The model under review builds one solid part; all positions refer to its coordinate system, in mm. A direction names the side the tool comes from. Round coordinates to 2 decimals unless told otherwise and drop trailing zeros. Loops run counter-clockwise (first coordinate to the right, second up) from the corner with the lowest first, then second, coordinate; pieces in that order, holes last. Notation, with made-up numbers: M 18.25,21 L 73.25,21 A26 cw 73.25,59 Z; hole C 30.5,-13 d3. An arc over 180 degrees is marked long. Use a Markdown table: item, result. Add a question column.
```python
from build123d import *

# Parameters (mm, degrees)
SKETCH1_W                    = 76.2
SKETCH1_H                    = 88.9
BOSS_EXTRUDE1_DEPTH          = 1.27
CUT_EXTRUDE_THIN1_DEPTH      = 59.599181735
CUT_EXTRUDE_THIN1_DEPTH_BACK = 2.794
SKETCH3_W                    = 2.794
SKETCH3_H                    = 44.704
CHAMFER1_SIZE                = 0.254


with BuildPart() as part:
    # Sketch1 → Boss-Extrude1 (new, symmetric)
    with BuildSketch(Plane(origin=(0, 0, 0), x_dir=(1, 0, 0), z_dir=(0, 1, 0))):
        Rectangle(SKETCH1_W, SKETCH1_H)
    extrude(amount=BOSS_EXTRUDE1_DEPTH, both=True)

    # Sketch3 → Cut-Extrude-Thin1 (cut, two sides: drawn at the far end of the back side and taken through both)
    with BuildSketch(Plane(origin=(0, 1.27, 0), x_dir=(1, 0, 0), z_dir=(0, 1, 0)).offset(-CUT_EXTRUDE_THIN1_DEPTH_BACK)):
        with Locations((0, -22.098)):
            Rectangle(SKETCH3_W, SKETCH3_H)
    extrude(amount=CUT_EXTRUDE_THIN1_DEPTH + CUT_EXTRUDE_THIN1_DEPTH_BACK, mode=Mode.SUBTRACT)

    # Chamfer1
    chamfer1_edges = [part.edges().sort_by_distance(p)[0] for p in [
        (38.1, 1.27, 0),
        (19.7485, -1.27, 44.45),
        (0, -1.27, -0.254),
        (1.397, -1.27, 22.098),
        (-1.397, -1.27, 22.098),
        (0, 1.27, -44.45),
        (19.7485, 1.27, 44.45),
        (1.397, 1.27, 22.098),
        (0, 1.27, -0.254),
        (-1.397, 1.27, 22.098),
        (-38.1, 1.27, 0),
        (0, -1.27, -44.45),
        (38.1, -1.27, 0),
        (-19.7485, -1.27, 44.45),
        (-38.1, -1.27, 0),
        (-19.7485, 1.27, 44.45),
    ]]
    chamfer(chamfer1_edges, length=CHAMFER1_SIZE)


solid = part.part
```
(1) To check wall thickness, follow probe 1 along X at (y, z) = (0.5, 30.5); probe 2 along X at (y, z) = (-1.1, 18); probe 3 along Z at (x, y) = (-0.5, -1.1). State the ranges of each line that lie inside material, in increasing order.
(2) Consider section B-B, the plane y = -0.1. Give the boundary of the cut face in (x, z).
(3) Consider section A-A, the plane z = 17. Give the boundary of the cut face in (x, y), then the cut area to 3 significant figures.
(4) For faces 1 (the face through (38.1, 0, 1)), 2 (the face through (-1.397, 0, 22)), list the 3-axis set-ups (+Z, -Z, +X, -X, +Y, -Y) from which the entire face can be reached by the end or side of a thin tool; tool diameter is ignored.
Found:
| question | item | result |
|---|---|---|
| 1 | probe 1 | x = -38.1 to -1.4, 1.4 to 38.1 |
| 1 | probe 2 | x = -38.02 to -1.48, 1.48 to 38.02 |
| 1 | probe 3 | z = -44.37 to -0.34 |
| 2 | outline | M -38.1,-44.45 L 38.1,-44.45 L 38.1,44.45 L 1.4,44.45 L 1.4,-0.25 L -1.4,-0.25 L -1.4,44.45 L -38.1,44.45 Z |
| 3 | outline | M -38.1,-1.02 L -37.85,-1.27 L -1.65,-1.27 L -1.4,-1.02 L -1.4,1.02 L -1.65,1.27 L -37.85,1.27 L -38.1,1.02 Z; M 1.4,-1.02 L 1.65,-1.27 L 37.85,-1.27 L 38.1,-1.02 L 38.1,1.02 L 37.85,1.27 L 1.65,1.27 L 1.4,1.02 Z |
| 3 | area | 186 mm^2 |
| 4 | face 1 | +Z, -Z, +X, +Y, -Y |
| 4 | face 2 | +Z, +Y, -Y |
